from build123d import *

# Parameters (mm, degrees)
SKETCH_1_W                  = 22
SKETCH_1_H                  = 39
EXTRUDE_1_DEPTH             = 4
SKETCH_2_W                  = 10
SKETCH_2_H                  = 1
CUT_EXTRUDE_1_DEPTH         = 40
SKETCH_3_R                  = 1.7
CUT_EXTRUDE_2_DEPTH         = 5
PATTERN_LINEAR_1_COUNT      = 2
PATTERN_LINEAR_1_PITCH      = 14
PATTERN_LINEAR_1_COUNT_DIR2 = 3
PATTERN_LINEAR_1_PITCH_DIR2 = 15.5


with BuildPart() as part:
    # 草圖1 → 填料-伸長1 (new body)
    with BuildSketch(Plane.XY):
        Rectangle(SKETCH_1_W, SKETCH_1_H)
    extrude(amount=EXTRUDE_1_DEPTH)

    # 草圖2 → 除料-伸長1 (cut, through all)
    with BuildSketch(Plane(origin=(0, 19.5, 0), x_dir=(1, 0, 0), z_dir=(0, 1, 0))):
        with Locations((0, -0.5)):
            Rectangle(SKETCH_2_W, SKETCH_2_H)
    extrude(amount=-CUT_EXTRUDE_1_DEPTH, mode=Mode.SUBTRACT)

    # 草圖3 → 除料-伸長2 (cut, through all)
    with BuildSketch(Plane(origin=(0, 0, 0), x_dir=(-1, 0, 0), z_dir=(0, 0, -1))):
        with Locations((-7, 15.5)):
            Circle(SKETCH_3_R)
    cut_extrude_2 = extrude(amount=-CUT_EXTRUDE_2_DEPTH, mode=Mode.SUBTRACT)

    # 直線複製排列1: Cut-Extrude 2 2 × 3
    with Locations(*[(-i * PATTERN_LINEAR_1_PITCH, -j * PATTERN_LINEAR_1_PITCH_DIR2, 0) for i in range(PATTERN_LINEAR_1_COUNT) for j in range(PATTERN_LINEAR_1_COUNT_DIR2) if (i, j) != (0, 0)]):
        add(cut_extrude_2, mode=Mode.SUBTRACT)


solid = part.part
Verification items for the finished model (mm, model axes). A direction names the side the tool comes from. Give positions to 0.01 mm unless a question says otherwise; leave off trailing zeros. Loops run counter-clockwise (first coordinate to the right, second up) from the corner with the lowest first, then second, coordinate; pieces in that order, holes last.
1. Release check for a two-part mould opening along Y. For faces 1 (the flat face through (0, 19.5, 2)), 2 (the flat face through (-9, 0, 0)), 3 (the cylindrical face through (8.7, -15.43, 1.97)) record: +Y half, -Y half, draft (parallel to the pull), parting line (faces both ways), or undercut.
Derived:
face 1: +Y half
face 2: draft
face 3: undercut
2. Material ranges on probe 1 along Y at (x, z) = (-7, 1.95); probe 2 along X at (y, z) = (1, 2.9); probe 3 along X at (y, z) = (5, 0.75), recorded low to high.
Derived:
probe 1: y = -19.5 to -17.2, -13.8 to -1.7, 1.7 to 13.8, 17.2 to 19.5
probe 2: x = -11 to -8.37, -5.63 to 5.63, 8.37 to 11
probe 3: x = -11 to -5, 5 to 11
3. Cross-section at D-D on x = 0.25. Record the cut outline in (y, z).
Derived:
outline: (-19.5, 1) - (19.5, 1) - (19.5, 4) - (-19.5, 4) - close
4. Cross-section at A-A on x = -7. Record the cut outline in (y, z).
Derived:
outline: (-19.5, 0) - (-17.2, 0) - (-17.2, 4) - (-19.5, 4) - close; (-13.8, 0) - (-1.7, 0) - (-1.7, 4) - (-13.8, 4) - close; (1.7, 0) - (13.8, 0) - (13.8, 4) - (1.7, 4) - close; (17.2, 0) - (19.5, 0) - (19.5, 4) - (17.2, 4) - close
5. Tool access check on faces 4 (the flat face through (0, 0, 4)), 5 (the flat face through (5, 0.3, 0.5)). Record the directions out of +Z, -Z, +X, -X, +Y, -Y that give a thin tool (end or side, any length) a straight path to the whole face; none if there is none.
Derived:
face 4: +Z, +X, -X, +Y, -Y
face 5: -Z, +Y, -Y
6. Cross-section at C-C on z = 2.3. Record the cut outline in (x, y), and give its area (3 significant figures).
Derived:
outline: (-11, -19.5) - (11, -19.5) - (11, 19.5) - (-11, 19.5) - close; hole circle Ø3.4 at (-7, -15.5); hole circle Ø3.4 at (-7, 0); hole circle Ø3.4 at (-7, 15.5); hole circle Ø3.4 at (7, -15.5); hole circle Ø3.4 at (7, 0); hole circle Ø3.4 at (7, 15.5)
area: 804 mm2
7. Cross-section at B-B on y = 0. Record the cut outline in (x, z), and give its area (3 significant figures).
Derived:
outline: (-11, 0) - (-8.7, 0) - (-8.7, 4) - (-11, 4) - close; (-5.3, 0) - (-5, 0) - (-5, 1) - (5, 1) - (5, 0) - (5.3, 0) - (5.3, 4) - (-5.3, 4) - close; (8.7, 0) - (11, 0) - (11, 4) - (8.7, 4) - close
area: 50.8 mm2
8. Go/stop test with a flat-tipped pin: P1, Ø2.5, axis at x = 7, y = -15.5, coming from the +Z side. Record where the tip stops, or that it passes through.
Derived:
P1: passes through
